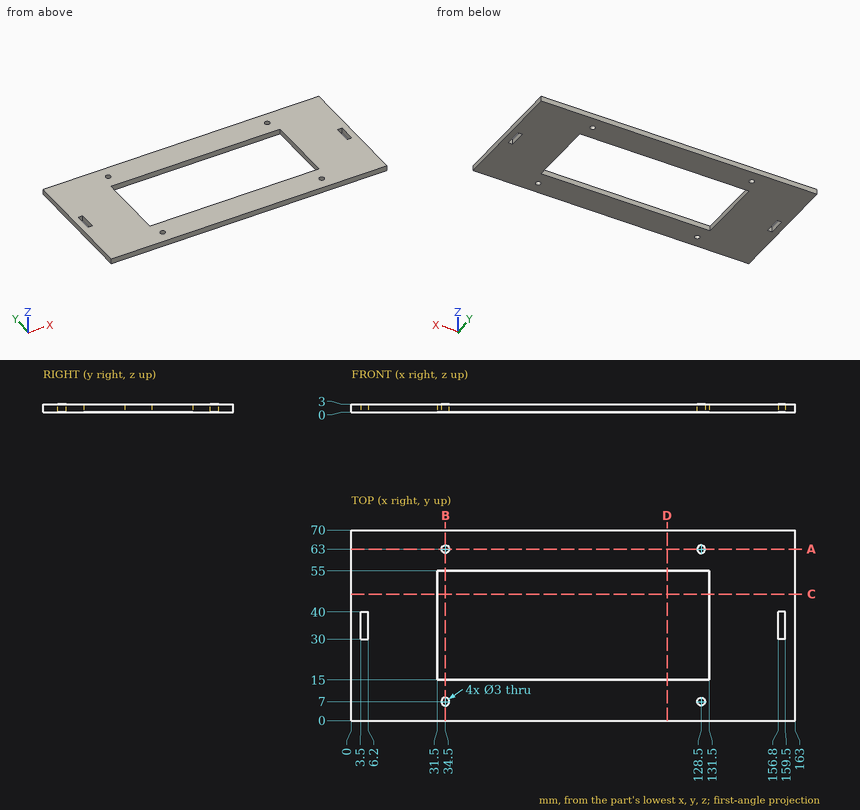
Can you work these out from the drawing? Everything is in mm from the part's minimum corner. Round coordinates to 2 decimals unless told otherwise and drop trailing zeros. Write each loop counter-clockwise with the first axis right and the second up, starting at its lowest first coordinate (ties: lowest second). Pieces come first, ordered by that corner, then holes. Notation, with made-up numbers: (5.25, 83) - (59.25, 83) arc R8 cw to (59.25, 90) - close; hole circle Ø7 at (-26.5, 53.25). An arc over 180 degrees is marked (long way). Write each question's results on one line, items separated by ' | '. Start each with the question number.
1) Suppose I cut it at D-D (x = 116). List the corners of the cut face in (y, z) for me.
2) Please list where these lines run through material, in increasing order: line 1 (X direction, y = 37.5, z = 2.2); line 2 (Y direction, x = 34.5, z = 2.05); line 3 (Y direction, x = 109, z = 1.9).
3) Suppose I cut it at A-A (y = 63). List the corners of the cut face in (x, z) for me.
4) Suppose I cut it at C-C (y = 46.5). List the corners of the cut face in (x, z) for me, and give its area (3 significant figures).
5) Suppose I cut it at B-B (x = 34.5). List the corners of the cut face in (y, z) for me, and give its area (3 significant figures).
Here are the results:
1) outline: (0, 0) - (15, 0) - (15, 3) - (0, 3) - close; (55, 0) - (70, 0) - (70, 3) - (55, 3) - close
2) line 1: x = 0 to 3.5, 6.2 to 31.5, 131.5 to 156.8, 159.5 to 163 | line 2: y = 0 to 5.5, 8.5 to 15, 55 to 61.5, 64.5 to 70 | line 3: y = 0 to 15, 55 to 70
3) outline: (0, 0) - (33, 0) - (33, 3) - (0, 3) - close; (36, 0) - (127, 0) - (127, 3) - (36, 3) - close; (130, 0) - (163, 0) - (163, 3) - (130, 3) - close
4) outline: (0, 0) - (31.5, 0) - (31.5, 3) - (0, 3) - close; (131.5, 0) - (163, 0) - (163, 3) - (131.5, 3) - close | area: 189 mm2
5) outline: (0, 0) - (5.5, 0) - (5.5, 3) - (0, 3) - close; (8.5, 0) - (15, 0) - (15, 3) - (8.5, 3) - close; (55, 0) - (61.5, 0) - (61.5, 3) - (55, 3) - close; (64.5, 0) - (70, 0) - (70, 3) - (64.5, 3) - close | area: 72.0 mm2
